Drawing for the job (mm, zero at the part's lowest x, y, z). A direction names the side the tool comes from. Coordinates: 2 decimals unless noted, no trailing zeros. Order: outer loops, then holes, each group sorted by start corner. A loop starts at its lowest first (then second) coordinate and runs counter-clockwise, first axis right, second up.
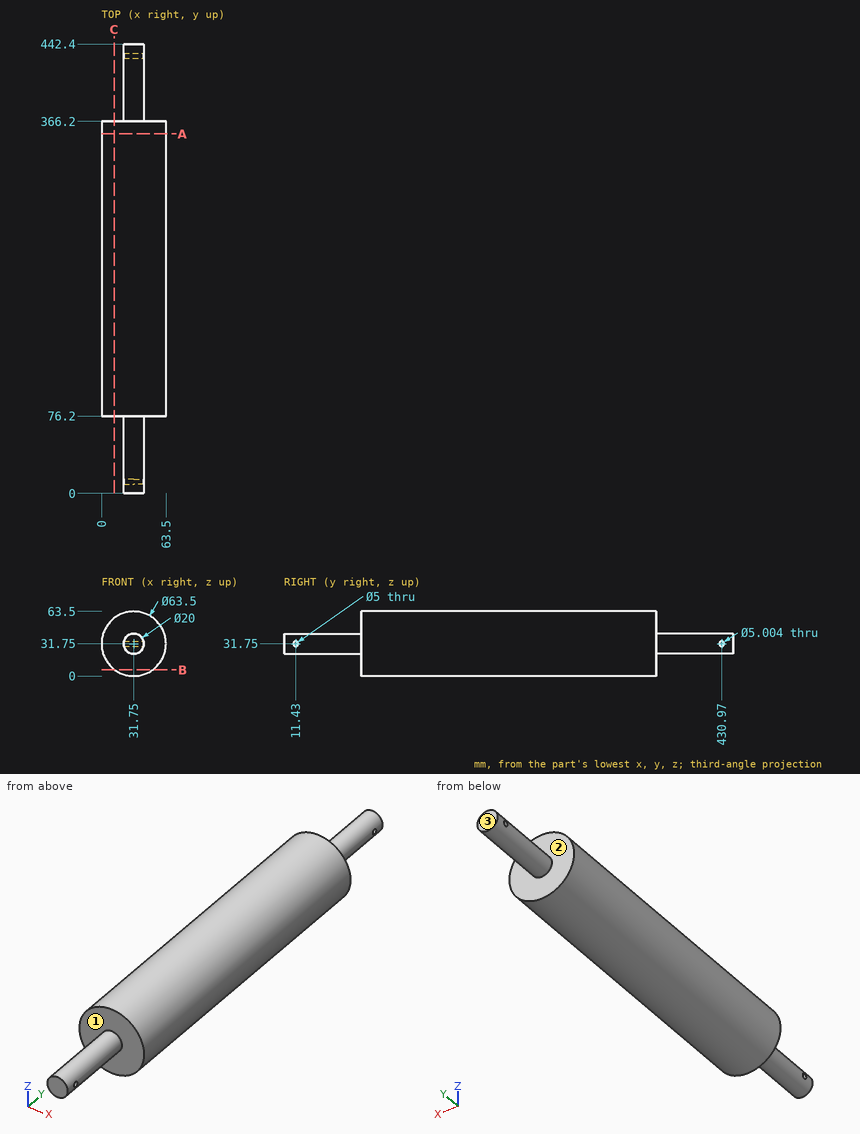
1) Slice it at A-A (y = 354). List the corners of the cut face in (x, z).
2) Slice it at C-C (x = 12.5). List the corners of the cut face in (y, z), plus the area to 3 significant figures.
3) Pin check, flat tips, straight feed: P1, Ø2, axis at x = 45.5, y = 358, coming from the +Z side; P2, Ø1, axis at x = 16.5, z = 50, coming from the +Y side; P3, Ø1.5, axis at y = 265.5, z = 39, coming from the +X side; P4, Ø4, axis at y = 11.43, z = 31.75, coming from the -X side. Stop position of each tip, or through.
4) Slice it at B-B (z = 6). List the corners of the cut face in (x, y).
5) Drill centre lines: probe 1 along Y at (x, z) = (34, 31.75); probe 2 along X at (y, z) = (201, 32); probe 3 along Z at (x, y) = (31, 430.97). Where is each one in solid material? Low to high.
6) Which spindle directions (+Z, -Z, +X, -X, +Y, -Y) get a long thin tool onto all of the face, cutting with end or side? Do the marked faces 1, 2 and 3. Say none if no direction does.
Worked out:
1. outline: circle Ø63.5 at (31.75, 31.75)
2. outline: (76.2, 6.5) - (366.2, 6.5) - (366.2, 57) - (76.2, 57) - close
2. area: 14,600 mm2
3. P1: stops at z = 60.83
3. P2: stops at y = 366.2
3. P3: stops at x = 62.83
3. P4: passes through
4. outline: (13.18, 76.2) - (50.32, 76.2) - (50.32, 366.2) - (13.18, 366.2) - close
5. probe 1: y = 0 to 8.93, 13.93 to 428.47, 433.47 to 442.4
5. probe 2: x = 0 to 63.5
5. probe 3: z = 21.78 to 29.25, 34.25 to 41.72
6. face 1: -Y
6. face 2: +Y
6. face 3: +Z, -Z, +X, -X, +Y
